Can you work these out from the model? Positions are in its coordinate system, mm. Face numbers are marked on the shaded views. A direction names the side the tool comes from. Coordinates: 2 decimals unless noted, no trailing zeros. Order: outer loops, then holes, each group sorted by start corner. A loop starts at its lowest first (then second) coordinate and runs counter-clockwise, first axis right, second up. Notation, with made-up numbers: (44.5, 71) -> (92.5, 71) arc R24 cw to (92.5, 90) -> close; hole circle Ø7 at (41.25, 22). An arc over 180 degrees is marked (long way). Use a Markdown table: item, result. Add a question column.
1. Suppose I cut it at A-A, the plane y = 12.5. State how many separate pieces and enclosed holes the cut face has, then the cut area to 3 significant figures.
2. If I drill on line 1 along Y through (x, z) = (31, -18), over which ranges is the centre line in solid material (lowest first)? Write a range as from..to.
3. Suppose I cut it at B-B, the plane x = 14. List the corners of the cut face in (y, z) for me.
4. For pin 1 Ø5 at (x, y) = (24, 11) entering from +Z; pin 2 Ø16 at (y, z) = (20.5, -29) entering from +X; pin 3 Ø9.5 at (y, z) = (20, -22.5) entering from -X; pin 4 Ø2.5 at (x, z) = (13.5, -15.5) entering from +Y, each with a flat end and sliding along its axis, tell me the tip position at first contact or that it passes through.
5. For the marked faces 1, 2 and 3, which set-ups out of +Z, -Z, +X, -X, +Y, -Y let a thin tool reach every point of the face, with its end or its side?
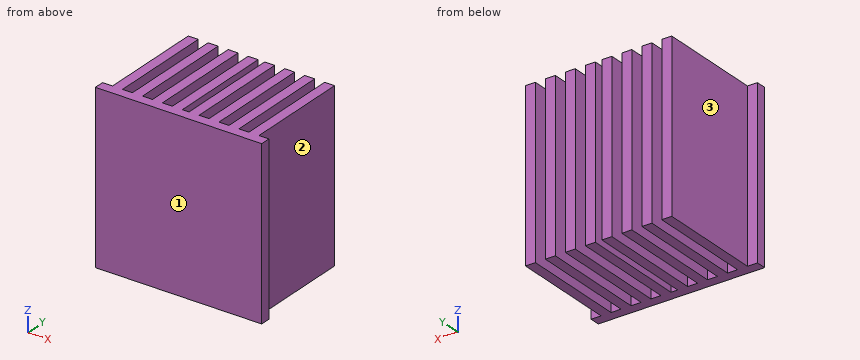
```python
from build123d import *

# Parameters (mm, degrees)
SKETCH2_W           = 50
SKETCH2_H           = 50
BOSS_EXTRUDE1_DEPTH = 3
SKETCH3_W           = 3
SKETCH3_H           = 50
BOSS_EXTRUDE2_DEPTH = 31.75


with BuildPart() as part:
    # Sketch2 → Boss-Extrude1 (new body)
    with BuildSketch(Plane(origin=(0, 0, 0), x_dir=(1, 0, 0), z_dir=(0, 1, 0))):
        with Locations((25, 25)):
            Rectangle(SKETCH2_W, SKETCH2_H)
    extrude(amount=BOSS_EXTRUDE1_DEPTH)

    # Sketch3 → Boss-Extrude2 (add)
    with BuildSketch(Plane(origin=(0, 3, 0), x_dir=(1, 0, 0), z_dir=(0, 1, 0))):
        with Locations((4.5, 25)):
            Rectangle(SKETCH3_W, SKETCH3_H)
        with Locations((10.5, 25)):
            Rectangle(SKETCH3_W, SKETCH3_H)
        with Locations((16.5, 25)):
            Rectangle(SKETCH3_W, SKETCH3_H)
        with Locations((22.5, 25)):
            Rectangle(SKETCH3_W, SKETCH3_H)
    boss_extrude2 = extrude(amount=BOSS_EXTRUDE2_DEPTH)

    # Mirror1: Boss-Extrude2 across plane
    add(boss_extrude2.mirror(Plane.ZY.offset(-25)))


solid = part.part
```
Worked out:
| question | item | result |
|---|---|---|
| 1 | separate pieces | 8 |
| 1 | enclosed holes | 0 |
| 1 | area | 1,200 mm² |
| 2 | line 1 | y = 0..3 |
| 3 | outline | (0, -50) -> (3, -50) -> (3, 0) -> (0, 0) -> close |
| 4 | pin 1 | stops at z = 0 |
| 4 | pin 2 | stops at x = 47 |
| 4 | pin 3 | stops at x = 3 |
| 4 | pin 4 | stops at y = 3 |
| 5 | face 1 | +Z, -Z, +X, -X, -Y |
| 5 | face 2 | +Z, -Z, +X, +Y |
| 5 | face 3 | +Z, -Z, -X, +Y |
